Source: CAD feature listing. Evaluate the final solid. Frame: model axes, mm. Coordinates: 2 decimals unless noted, no trailing zeros. Order: outer loops, then holes, each group sorted by start corner. A loop starts at its lowest first (then second) coordinate and runs counter-clockwise, first axis right, second up. Notation, with made-up numbers: (78, -18.5) -> (117, -18.5) arc R38 cw to (117, 20.5) -> close; hole circle Ø2 at (70.5, 28). An arc over 180 degrees is marked (long way). Write item = value, one per line. Start each with the question number.
Item 1: Section query C-C (y = 3.4). Count the separate pieces of the cut face and the enclosed holes in it, then the cut area to 3 significant figures.
Item 2: Section query D-D (z = 30). Output: boundary loops of the cut face in (x, y), then the cut area to 3 significant figures.
Item 3: Contact query for flat-ended pins moving along their axis: pin 1 (1 mm diameter, centred on y = 0.5, z = 28.5, fed in from +X); pin 2 (8 mm diameter, centred on x = 0, z = -10, fed in from -Y); pin 3 (2 mm diameter, centred on x = -11, y = 2.5, fed in from -Z); pin 4 (2 mm diameter, centred on y = 1, z = -21, fed in from +X). Output: stop coordinate, or through.
Item 4: Ray query, line 1 along Z through (x, y) = (0, 1.4); line 2 along Z through (x, y) = (-28, 2.55); line 3 along Z through (x, y) = (27, 1.45). Return the intervals inside material, ascending. Write a range as [from, to].
Item 5: Section query A-A (x = 0). Output: boundary loops of the cut face in (y, z), then the cut area to 3 significant figures.
Item 6: Section query B-B (z = -14). Output: boundary loops of the cut face in (x, y).
Autodesk Inventor part; units mm, degrees
ref_plane "YZ Plane" through (0, 0, 0) normal (1, 0, 0) x (0, 1, 0)
ref_plane "XZ Plane" through (0, 0, 0) normal (0, 1, 0) x (-1, 0, 0)
ref_plane "XY Plane" through (0, 0, 0) normal (0, 0, 1) x (1, 0, 0)
sketch "Sketch1" plane through (0, 0, 0) normal (0, 1, 0) x (-1, 0, 0)
  circle A0 centre (0, 0) radius 42.5
  line L0 (0, 0) -> (0, -5)
  line L1 (0, 0) -> (0, 5)
  circle A1 centre (28, 10) radius 5
  circle A2 centre (0, 10) radius 5
  circle A3 centre (-28, 10) radius 5
  circle A4 centre (28, -10) radius 5
  circle A5 centre (-28, -10) radius 5
  circle A6 centre (0, -10) radius 5
  circle A7 centre (0, 30) radius 5
  circle A8 centre (0, -30) radius 5
  dimension "d2" = 85
  dimension "d5" = 10
  dimension "d6" = 10
  dimension "d7" = 10
  dimension "d10" = 10
  dimension "d11" = 10
  dimension "d12" = 10
  dimension "d13" = 10
  dimension "d15" = 10
extrude "Extrusion1" add sketch "Sketch1" along normal blind 4
properties part number "Wires_Base"
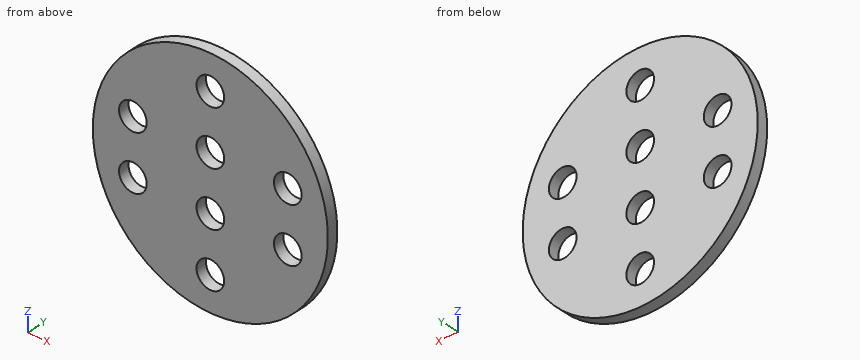
Computed:
q1.separate_pieces = 1
q1.enclosed_holes = 8
q1.area = 5,050 mm^2
q2.outline = (-30.1, 0) -> (-5, 0) -> (-5, 4) -> (-30.1, 4) -> close; (5, 0) -> (30.1, 0) -> (30.1, 4) -> (5, 4) -> close
q2.area = 201 mm^2
q3.pin_1 = 31.97
q3.pin_2 = through
q3.pin_3 = -41.31
q3.pin_4 = 37.5
q4.line_1 = [-42.5, -35], [-25, -15], [-5, 5], [15, 25], [35, 42.5]
q4.line_2 = [-31.97, -15], [-5, 5], [15, 31.97]
q4.line_3 = [-32.82, -14.9], [-5.1, 5.1], [14.9, 32.82]
q5.outline = (0, -42.5) -> (4, -42.5) -> (4, -35) -> (0, -35) -> close; (0, -25) -> (4, -25) -> (4, -15) -> (0, -15) -> close; (0, -5) -> (4, -5) -> (4, 5) -> (0, 5) -> close; (0, 15) -> (4, 15) -> (4, 25) -> (0, 25) -> close; (0, 35) -> (4, 35) -> (4, 42.5) -> (0, 42.5) -> close
q5.area = 180 mm^2
q6.outline = (-40.13, 0) -> (-31, 0) -> (-31, 4) -> (-40.13, 4) -> close; (-25, 0) -> (-3, 0) -> (-3, 4) -> (-25, 4) -> close; (3, 0) -> (25, 0) -> (25, 4) -> (3, 4) -> close; (31, 0) -> (40.13, 0) -> (40.13, 4) -> (31, 4) -> close
